```python
from build123d import *

# Parameters (mm, degrees)
F0_W      = 101.6
F0_H      = 38.1
F1_DEPTH  = 127
F2_W      = 50.8
F2_H      = 12.7
F1_FACE_W = 101.6
F1_FACE_H = 38.1
F3_DEPTH  = 25.4
F4_T      = -2.54


with BuildPart() as f1:
    # F0 (on Front) → F1 (new body)
    with BuildSketch(Plane.XZ):
        Rectangle(F0_W, F0_H)
    extrude(amount=F1_DEPTH)

    # F2 (on Front) + F1_face (on face) → F3 (join)
    with BuildSketch(Plane.XZ):
        Rectangle(F2_W, F2_H)
    with BuildSketch(Plane.XZ.offset(127)):
        Rectangle(F1_FACE_W, F1_FACE_H)
    extrude(amount=-F3_DEPTH)

    # F4
    f4_openings = [f1.faces().sort_by_distance(p)[0] for p in [
        (0, -63.5, 19.05),
    ]]
    offset(amount=F4_T, openings=f4_openings, kind=Kind.INTERSECTION)


solid = f1.part
```
Work out the finished part from the listing and answer in its coordinate system (mm). A direction names the side the tool comes from. Give positions to 0.01 mm unless a question says otherwise; leave off trailing zeros. Loops run counter-clockwise (first coordinate to the right, second up) from the corner with the lowest first, then second, coordinate; pieces in that order, holes last. Notation, with made-up numbers: (49.5, 5.25) - (87.5, 5.25) arc R12 ccw to (87.5, 26.25) - close; hole circle Ø4 at (-38, 8.5). An arc over 180 degrees is marked (long way). One line per question, with ' | ' between items.
(1) The part is cut by section D-D (x = 42). Write down the section's boundary in (y, z).
Recorded:
outline: (-127, -19.05) - (0, -19.05) - (0, 19.05) - (-2.54, 19.05) - (-2.54, -16.51) - (-124.46, -16.51) - (-124.46, 19.05) - (-127, 19.05) - close
(2) The mould has two halves that part along X. Classify faces 1 (the face through (0, -2, 19.05)), 2 (the face through (0, 10, 3.81)), 3 (the face through (-50.8, -63, 0)): +X half, -X half, draft (parallel to the pull), parting line (faces both ways), or undercut.
Recorded:
face 1: draft | face 2: undercut | face 3: -X half
(3) The part is cut by section C-C (y = -109.5). Write down the section's boundary in (x, z).
Recorded:
outline: (-50.8, -19.05) - (50.8, -19.05) - (50.8, 19.05) - (48.26, 19.05) - (48.26, -16.51) - (-48.26, -16.51) - (-48.26, 19.05) - (-50.8, 19.05) - close
(4) Each of these flat-tipped pins is pushed along its axis until it touches: pin 1 Ø1 at (x, y) = (38.5, -19) entering from +Z; pin 2 Ø8 at (x, z) = (32, -1.5) entering from +Y; pin 3 Ø10 at (y, z) = (14.5, 1) entering from +X. Where does it stop, or does it pass through?
Recorded:
pin 1: stops at z = -16.51 | pin 2: stops at y = 0 | pin 3: stops at x = 25.4
(5) Straight lines are drawn through the part: probe 1 along X at (y, z) = (-85, -1.5); probe 2 along Y at (x, z) = (24.5, 3); probe 3 along Y at (x, z) = (21.5, -1). For each, find the intervals that lie inside material, in ascending order.
Recorded:
probe 1: x = -50.8 to -48.26, 48.26 to 50.8 | probe 2: y = -127 to -124.46, -2.54 to 25.4 | probe 3: y = -127 to -124.46, 22.86 to 25.4
(6) The part is cut by section B-B (x = 5). Write down the section's boundary in (y, z).
Recorded:
outline: (-127, -19.05) - (0, -19.05) - (0, -6.35) - (25.4, -6.35) - (25.4, 6.35) - (0, 6.35) - (0, 19.05) - (-2.54, 19.05) - (-2.54, 3.81) - (22.86, 3.81) - (22.86, -3.81) - (-2.54, -3.81) - (-2.54, -16.51) - (-124.46, -16.51) - (-124.46, 19.05) - (-127, 19.05) - close
(7) The part is cut by section A-A (z = -8). Write down the section's boundary in (x, y), then the cut area to 3 significant figures.
Recorded:
outline: (-50.8, -127) - (50.8, -127) - (50.8, 0) - (-50.8, 0) - close; hole (-48.26, -124.46) - (48.26, -124.46) - (48.26, -2.54) - (-48.26, -2.54) - close | area: 1,140 mm²
(8) A tool of negligible diameter and unlimited length cuts with its end or side. For faces 4 (the face through (-1, -2.54, 5)), 5 (the face through (0, 22.86, 0)), 6 (the face through (0, 13, -6.35)), from which of +Z, -Z, +X, -X, +Y, -Y can it reach the whole face along a straight path? Write none if from no direction.
Recorded:
face 4: +Z | face 5: none | face 6: -Z, +X, -X, +Y
